Design review of the part shown in the three views and the two pictorial views. Dimensions are in mm from the part's minimum x, y and z. Coordinates: 2 decimals unless noted, no trailing zeros. Loops run counter-clockwise (first coordinate to the right, second up) from the corner with the lowest first, then second, coordinate; pieces in that order, holes last. Notation, with made-up numbers: (45.5, -18.5) -> (50.5, -18.5) arc R27 ccw to (50.5, 0.5) -> close; hole circle Ø7 at (39, -11.5). An arc over 180 degrees is marked (long way). One line per item, written item: value.
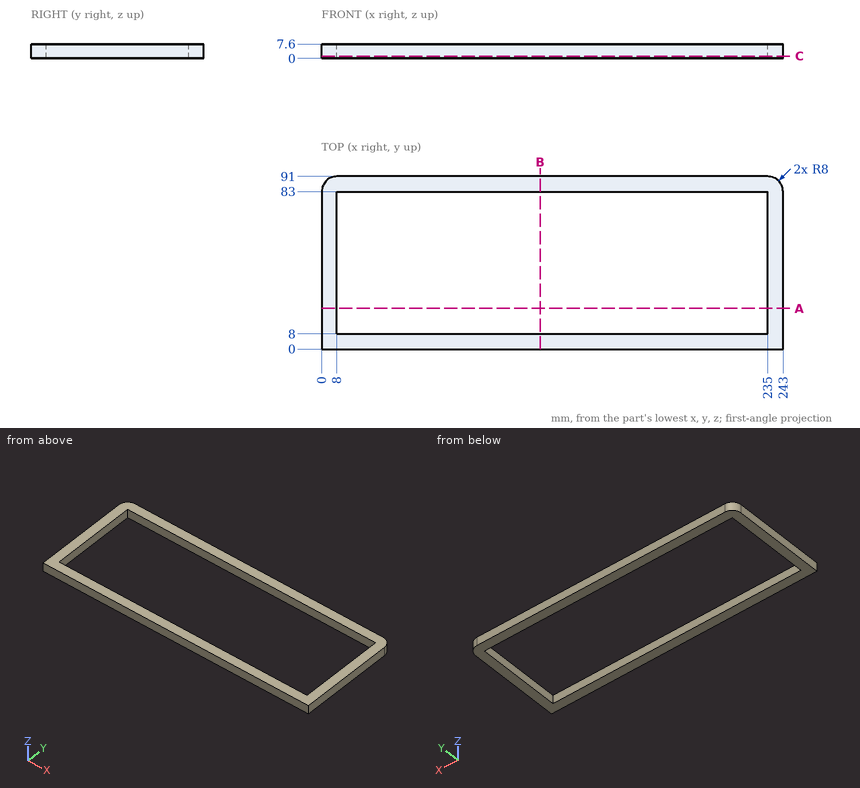
1. Take a section at B-B, the plane x = 115. Give the boundary of the cut face in (y, z), and give its area (3 significant figures).
Return value:
outline: (0, 0) -> (8, 0) -> (8, 7.6) -> (0, 7.6) -> close; (83, 0) -> (91, 0) -> (91, 7.6) -> (83, 7.6) -> close
area: 122 mm2
2. Take a section at A-A, the plane y = 21.5. Give the boundary of the cut face in (x, z), and give its area (3 significant figures).
Return value:
outline: (0, 0) -> (8, 0) -> (8, 7.6) -> (0, 7.6) -> close; (235, 0) -> (243, 0) -> (243, 7.6) -> (235, 7.6) -> close
area: 122 mm2
3. Take a section at C-C, the plane z = 1.25. Give the boundary of the cut face in (x, y), and give its area (3 significant figures).
Return value:
outline: (0, 0) -> (243, 0) -> (243, 83) arc R8 ccw to (235, 91) -> (8, 91) arc R8 ccw to (0, 83) -> close; hole (8, 8) -> (235, 8) -> (235, 83) -> (8, 83) -> close
area: 5,060 mm2
4. To check wall thickness, follow probe 1 along Y at (x, z) = (204, 4.5); probe 2 along X at (y, z) = (59, 5); probe 3 along X at (y, z) = (86, 7). State the ranges of each line that lie inside material, in increasing order. Write a range as from..to.
Return value:
probe 1: y = 0..8, 83..91
probe 2: x = 0..8, 235..243
probe 3: x = 0.58..242.42
5. Insertion check: pin 1 Ø4 at (x, z) = (131.5, 6) entering from -Y. The pin has a flat end and moves straight along its axis. Give the tip position at first contact, or say it passes through.
Return value:
pin 1: stops at y = 0
